Could you check a few things on this model? Use its own coordinates, in mm. A direction names the side the tool comes from. Give positions to 0.01 mm unless a question says otherwise; leave off trailing zeros. Loops run counter-clockwise (first coordinate to the right, second up) from the corner with the lowest first, then second, coordinate; pieces in that order, holes last. Notation, with made-up numbers: (15, 10.25) -> (57, 10.25) arc R20 cw to (57, 18.25) -> close; hole circle Ø1 at (27, 38). An arc over 180 degrees is marked (long way). Put each result on its own line as item: value.
```python
from build123d import *

# Parameters (mm, degrees)
CROQUIS1_R              = 10
SALIENTE_EXTRUIR1_DEPTH = 23
CHAFL_N1_SIZE           = 2
CROQUIS2_R              = 8.5
CORTAR_EXTRUIR1_DEPTH   = 15


with BuildPart() as part:
    # Croquis1 → Saliente-Extruir1 (new body)
    with BuildSketch(Plane.XY):
        Circle(CROQUIS1_R)
    extrude(amount=-SALIENTE_EXTRUIR1_DEPTH)

    # Chaflán1
    chafl_n1_edges = [part.edges().sort_by_distance(p)[0] for p in [
        (-10, 0, -23),
    ]]
    chamfer(chafl_n1_edges, length=CHAFL_N1_SIZE)

    # Croquis2 → Cortar-Extruir1 (cut)
    with BuildSketch(Plane.XY):
        Circle(CROQUIS2_R)
    extrude(amount=-CORTAR_EXTRUIR1_DEPTH, mode=Mode.SUBTRACT)


solid = part.part
```
1. I need wall thicknesses on line 1 (Y direction, x = 0, z = -8.25); line 2 (X direction, y = 6.5, z = -10.25); line 3 (Y direction, x = 4.75, z = -7.5). Which ranges of each line are inside material? Lowest first, please.
Recorded:
line 1: y = -10 to -8.5, 8.5 to 10
line 2: x = -7.6 to -5.48, 5.48 to 7.6
line 3: y = -8.8 to -7.05, 7.05 to 8.8
2. Thinking about a two-plate mould opening in Y: for faces 1 (the face through (0, 0, -23)), 2 (the face through (-2.17, -9.76, -10.35)), 3 (the face through (0, 0, -15)), which applies, pulls with the +Y half, pulls with the -Y half, needs draft (parallel to the pull), parting line crosses it, or undercut?
Recorded:
face 1: needs draft
face 2: parting line crosses it
face 3: undercut
3. If we section it at C-C (z = -13.5): List the corners of the cut face in (x, y) for me, then the cut area to 3 significant figures.
Recorded:
outline: circle Ø20 at (0, 0); hole circle Ø17 at (0, 0)
area: 87.2 mm^2
4. If we section it at A-A (x = 0): List the corners of the cut face in (y, z) for me, then the cut area to 3 significant figures.
Recorded:
outline: (-10, -21) -> (-8, -23) -> (8, -23) -> (10, -21) -> (10, 0) -> (8.5, 0) -> (8.5, -15) -> (-8.5, -15) -> (-8.5, 0) -> (-10, 0) -> close
area: 201 mm^2
5. If we section it at D-D (z = -19.25): List the corners of the cut face in (x, y) for me.
Recorded:
outline: circle Ø20 at (0, 0)
6. I'm going to push flat-ended pins straight in: pin 1 (4 mm diameter, centred on x = 7, y = 0.5, fed in from +Z); pin 2 (4 mm diameter, centred on x = 7, z = -17, fed in from +Y); pin 3 (6 mm diameter, centred on x = -7.5, z = -18, fed in from -Y); pin 4 (5 mm diameter, centred on x = -4, y = -3, fed in from +Z). Where does each tip first touch, or does it pass through?
Recorded:
pin 1: stops at z = 0
pin 2: stops at y = 8.66
pin 3: stops at y = -8.93
pin 4: stops at z = -15
7. For faces 4 (the face through (4.57, 7.167, -7.395)), 5 (the face through (-4.5, -7.4, 0)), which set-ups out of +Z, -Z, +X, -X, +Y, -Y let a thin tool reach every point of the face, with its end or its side?
Recorded:
face 4: +Z
face 5: +Z, +X, -X, +Y, -Y
